Verification items for the finished model (mm, model axes). Face numbers are marked on the shaded views. A direction names the side the tool comes from. Round coordinates to 2 decimals unless told otherwise and drop trailing zeros. Write each loop counter-clockwise with the first axis right and the second up, starting at its lowest first coordinate (ties: lowest second). Pieces come first, ordered by that corner, then holes. Notation, with made-up numbers: (2.5, 48.5) - (53.5, 48.5) arc R27 cw to (53.5, 69.5) - close; hole circle Ø8 at (88, -38.75). An arc over 180 degrees is marked (long way). Answer as a JSON object with one key per item and string values.
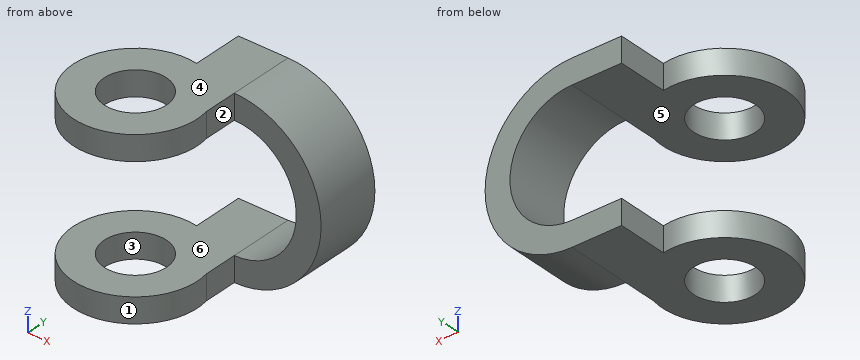
```python
from build123d import *

# Parameters (mm, degrees)
SKETCH1_R           = 12.5
BOSS_EXTRUDE1_DEPTH = 5
SKETCH2_R           = 12.5
BOSS_EXTRUDE2_DEPTH = 5
SKETCH4_W           = 10
SKETCH4_H           = 20
BOSS_EXTRUDE4_DEPTH = 5
SKETCH5_W           = 10
SKETCH5_H           = 20
BOSS_EXTRUDE5_DEPTH = 5
SKETCH8_R           = 6.25
CUT_EXTRUDE2_DEPTH  = 35
SKETCH12_W          = 5
SKETCH12_H          = 13.195782459


with BuildPart() as part:
    # Sketch1 → Boss-Extrude1 (new body)
    with BuildSketch(Plane.XY):
        Circle(SKETCH1_R)
    extrude(amount=BOSS_EXTRUDE1_DEPTH)

    # Sketch4 → Boss-Extrude4 (add)
    with BuildSketch(Plane.XY.offset(5)):
        with Locations((7.235331181, 12.5586463)):
            Rectangle(SKETCH4_W, SKETCH4_H)
    extrude(amount=-BOSS_EXTRUDE4_DEPTH)


with BuildPart() as body_2:
    # Sketch2 → Boss-Extrude2 (new body)
    with BuildSketch(Plane.XY.offset(30)):
        Circle(SKETCH2_R)
    extrude(amount=BOSS_EXTRUDE2_DEPTH)

    # Sketch5 → Boss-Extrude5 (add)
    with BuildSketch(Plane(origin=(0, 0, 30), x_dir=(-1, 0, 0), z_dir=(0, 0, -1))):
        with Locations((-7.235331181, 12.5586463)):
            Rectangle(SKETCH5_W, SKETCH5_H)
    extrude(amount=-BOSS_EXTRUDE5_DEPTH)


with BuildPart() as cut_extrude2_tool:
    # Sketch8 → Cut-Extrude2 (new body)
    with BuildSketch(Plane(origin=(0, 0, 0), x_dir=(-1, 0, 0), z_dir=(0, 0, -1))):
        Circle(SKETCH8_R)
    extrude(amount=-CUT_EXTRUDE2_DEPTH)


with BuildPart() as part_1:
    add(part.part)

    # Cut-Extrude2: cut by cut_extrude2_tool
    add(cut_extrude2_tool.part, mode=Mode.SUBTRACT)



with BuildPart() as body_2_1:
    add(body_2.part)

    # Cut-Extrude2: cut by cut_extrude2_tool
    add(cut_extrude2_tool.part, mode=Mode.SUBTRACT)


with BuildPart() as part_2:
    add(part_1.part)

    add(body_2_1.part)  # Sweep2 merges body 2
    # Sweep2: sweep along a path in Sketch14
    with BuildLine(Plane(origin=(0, 15.960755071, 0), x_dir=(1, 0, 0), z_dir=(0, 1, 0))) as sweep2_path:
        ThreePointArc((12.235331181, -32.5), (27.235331181, -17.5), (12.235331181, -2.5))
    # Sketch12 → Sweep2 (sweep)
    with BuildSketch(Plane(origin=(12.235331181, 0, 0), x_dir=(0, 0, -1), z_dir=(1, 0, 0))):
        with Locations((-32.5, 15.960755071)):
            Rectangle(SKETCH12_W, SKETCH12_H)
    sweep(path=sweep2_path.line)


solid = part_2.part
```
1. Access from +Z, -Z, +X, -X, +Y, -Y to the whole of each face (thin tool, end or side, straight path). Record for the marked faces 1 and 2.
Completed:
{"face 1": "+Z, -Z", "face 2": "+Z, -Z, +X"}
2. Cross-section at D-D (x = 11.5). Record the boundary of the cut face in (y, z), plus the area to 3 significant figures.
Completed:
{"outline": "(-4.9, 0) - (22.56, 0) - (22.56, 5) - (-4.9, 5) - close; (-4.9, 30) - (22.56, 30) - (22.56, 35) - (-4.9, 35) - close", "area": "275 mm^2"}
3. Material ranges on probe 1 along Z at (x, y) = (-2, -10); probe 2 along Y at (x, z) = (0, 2.2); probe 3 along Y at (x, z) = (26.5, 10.5), recorded low to high. Write a range as from..to.
Completed:
{"probe 1": "z = 0..5, 30..35", "probe 2": "y = -12.5..-6.25, 6.25..12.5", "probe 3": "y = 9.36..22.56"}
4. Go/stop test with flat-tipped pins: pin 1 (4 mm diameter, centred on y = 9.5, z = 27.5, fed in from +X); pin 2 (4 mm diameter, centred on y = 16, z = 2.5, fed in from -X); pin 3 (2 mm diameter, centred on x = 12, z = 31.5, fed in from -Y). Record where each tip stops, or that it passes through.
Completed:
{"pin 1": "stops at x = 27.8", "pin 2": "stops at x = 2.24", "pin 3": "stops at y = -5.94"}
5. Mould release check, pull along Z, two halves, no side actions. Record for the marked faces 3, 4, 5 and 6: released by +Z, released by -Z, zero draft, split by the parting line, or undercut.
Completed:
{"face 3": "zero draft", "face 4": "released by +Z", "face 5": "undercut", "face 6": "undercut"}
6. Cross-section at A-A (x = 0). Record the boundary of the cut face in (y, z).
Completed:
{"outline": "(-12.5, 0) - (-6.25, 0) - (-6.25, 5) - (-12.5, 5) - close; (-12.5, 30) - (-6.25, 30) - (-6.25, 35) - (-12.5, 35) - close; (6.25, 0) - (12.5, 0) - (12.5, 5) - (6.25, 5) - close; (6.25, 30) - (12.5, 30) - (12.5, 35) - (6.25, 35) - close"}
7. Cross-section at B-B (y = -8). Record the boundary of the cut face in (x, z).
Completed:
{"outline": "(-9.6, 0) - (9.6, 0) - (9.6, 5) - (-9.6, 5) - close; (-9.6, 30) - (9.6, 30) - (9.6, 35) - (-9.6, 35) - close"}
